Drawing for the job (mm, zero at the part's lowest x, y, z). A direction names the side the tool comes from. Give positions to 0.01 mm unless a question says otherwise; leave off trailing zeros. Loops run counter-clockwise (first coordinate to the right, second up) from the corner with the lowest first, then second, coordinate; pieces in that order, holes last. Notation, with made-up numbers: M 86,-2 L 139,-2 A9 cw 139,3 Z; hole C 59.5,60.5 d4. An arc over 180 degrees is marked long. Answer in a Markdown table with one row per item. Add a question column.
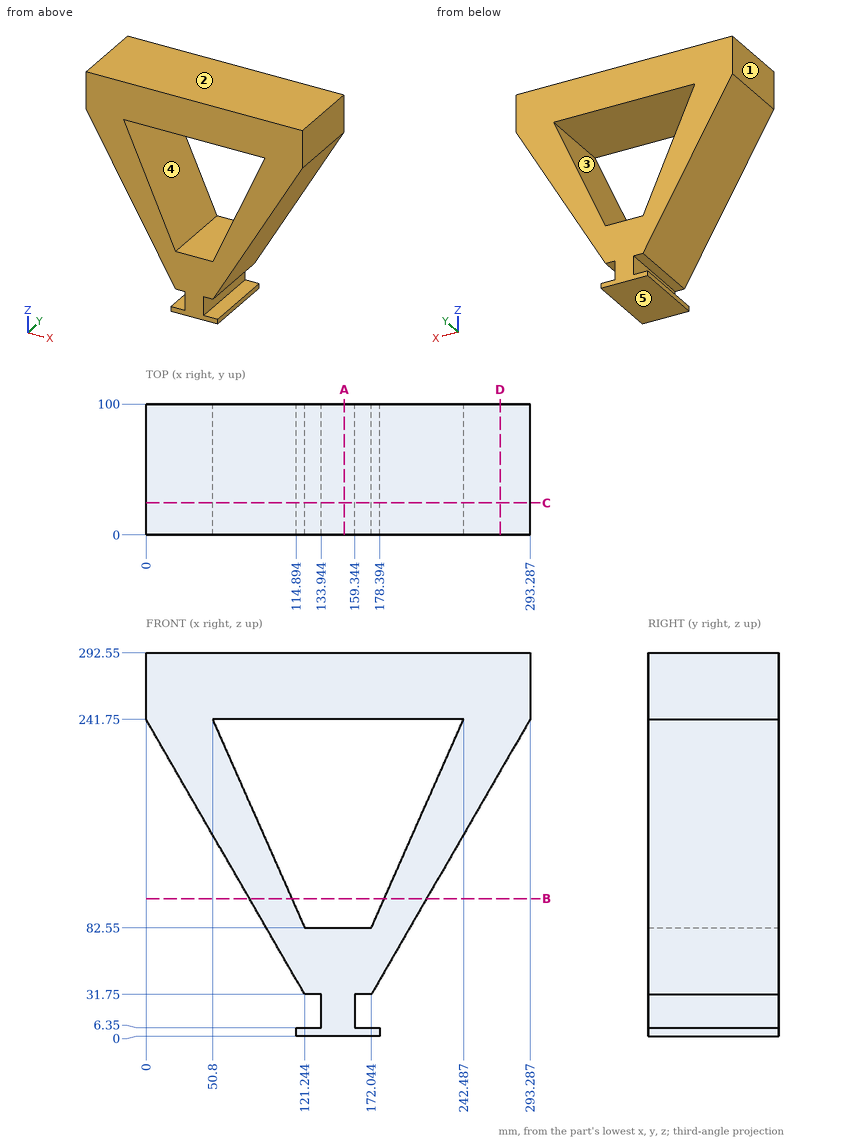
(1) Slice it at C-C, the plane y = 24.5. Give the cut face in (x, z), then the cut area to 3 significant figures.
(2) Slice it at D-D, the plane x = 270.5. Give the cut face in (y, z).
(3) Pull direction Z, two halves, no side cores. Call the marked faces 1, 2 and 3: +Z half, -Z half, draft (parallel to the pull), parting line (faces both ways), or undercut.
(4) Slice it at B-B, the plane z = 105. Give the cut face in (x, y) (1 decimal), then the cut area to 3 significant figures.
(5) Pin check, flat tips, straight feed: pin 1 (6.5 mm diameter, centred on x = 129, y = 48.5, fed in from -Z); pin 2 (5 mm diameter, centred on y = 54, z = 40, fed in from +X); pin 3 (1.5 mm diameter, centred on y = 78, z = 71, fed in from +X); pin 4 (5 mm diameter, centred on y = 60.5, z = 234, fed in from +X) (1 decimal). Stop position of each tip, or through.
(6) Wall check: line 1 (Z direction, x = 143, y = 63.5); line 2 (X direction, y = 36.5, z = 102.5) (1 decimal); line 3 (X direction, y = 52.5, z = 199.5) (1 decimal). Give the ranges that are in metal, low to high.
(7) Slice it at A-A, the plane x = 151.5. Give the cut face in (y, z).
(8) Tool access for the marked faces 4 and 5: list every direction of +Z, -Z, +X, -X, +Y, -Y with a clear straight run to the whole face (end or side of a thin tool).
Solution:
| question | item | result |
|---|---|---|
| 1 | outline | M 0,241.75 L 121.24,31.75 L 133.94,31.75 L 133.94,6.35 L 114.89,6.35 L 114.89,0 L 178.39,0 L 178.39,6.35 L 159.34,6.35 L 159.34,31.75 L 172.04,31.75 L 293.29,241.75 L 293.29,292.55 L 0,292.55 Z; hole M 50.8,241.75 L 121.24,82.55 L 172.04,82.55 L 242.49,241.75 Z |
| 1 | area | 32,800 mm^2 |
| 2 | outline | M 0,202.28 L 100,202.28 L 100,292.55 L 0,292.55 Z |
| 3 | face 1 | draft |
| 3 | face 2 | +Z half |
| 3 | face 3 | undercut |
| 4 | outline | M 79,0 L 111.3,0 L 111.3,100 L 79,100 Z; M 182,0 L 214.3,0 L 214.3,100 L 182,100 Z |
| 4 | area | 6,470 mm^2 |
| 5 | pin 1 | z = 0 |
| 5 | pin 2 | x = 178.25 |
| 5 | pin 3 | x = 195.14 |
| 5 | pin 4 | x = 290.3 |
| 6 | line 1 | 0 to 82.55, 241.75 to 292.55 |
| 6 | line 2 | 80.4 to 112.4, 180.9 to 212.9 |
| 6 | line 3 | 24.4 to 69.5, 223.8 to 268.9 |
| 7 | outline | M 0,0 L 100,0 L 100,82.55 L 0,82.55 Z; M 0,241.75 L 100,241.75 L 100,292.55 L 0,292.55 Z |
| 8 | face 4 | +Y, -Y |
| 8 | face 5 | -Z, +X, -X, +Y, -Y |
